The listing builds one solid part. Answer for the finished solid, in the listing's coordinates (mm). A direction names the side the tool comes from. Give positions to 0.01 mm unless a question says otherwise; leave off trailing zeros. Write each loop counter-clockwise with the first axis right and the second up, starting at its lowest first coordinate (ties: lowest second). Pieces come first, ordered by that corner, then holes. Notation, with made-up numbers: (-24.75, 46.5) - (9.25, 46.5) arc R17 cw to (9.25, 64.5) - close; hole circle Ø10 at (-4, 25.25). An arc over 180 degrees is marked (long way). Answer as CSV lines item,"result". Start each with the question number.
(1) For a pull along X with two mould halves and no side action, classify faces 5 (the face through (2, 3, 0)), 6 (the face through (20, 2, 0)), 7 (the face through (10, 0, 0)) as pulls with the +X half, pulls with the -X half, needs draft (parallel to the pull), parting line crosses it, or undercut.
(2) Straight lines are drawn through the part: probe 1 along X at (y, z) = (2.5, 0.8); probe 2 along Y at (x, z) = (2.75, 0.45); probe 3 along Z at (x, y) = (1.5, 5.2). For each, find the intervals that lie inside material, in ascending order.
(3) Find section C-C (x = 7.5). Write down the section's boundary in (y, z).
(4) Find section D-D (y = 2.7). Write down the section's boundary in (x, z).
(5) Each of these flat-tipped pins is pushed along its axis until it touches: pin 1 Ø1 at (y, z) = (4, 0.5) entering from -X; pin 2 Ø0.8 at (x, z) = (19.5, -1.5) entering from +Y; pin 3 Ø0.8 at (x, y) = (1, 4.5) entering from +Z; pin 4 Ø1.2 at (x, y) = (19, 5) entering from -Z. Where does it stop, or does it pass through?
(6) Find section B-B (z = 0.15). Write down the section's boundary in (x, y).
(7) For faces 1 (the face through (1, 4, 1.5)), 2 (the face through (18, 3, 0)), 3 (the face through (1, 5, -1)), 4 (the face through (10, 1, 2)), determine the directions among +Z, -Z, +X, -X, +Y, -Y from which every point of the face is accessible in a straight line to the end or side of a thin tool.
(8) Find section A-A (y = 5.1). Write down the section's boundary in (x, z), then the cut area to 3 significant figures.
from build123d import *

# Parameters (mm, degrees)
BOSS_EXTRUDE1_DEPTH      = 2
BOSS_EXTRUDE1_DEPTH_BACK = 2
SKETCH2_W                = 1
SKETCH2_H                = 1.5
CUT_EXTRUDE1_DEPTH       = 21.838665984


with BuildPart() as part:
    # Sketch1 → Boss-Extrude1 (new, two sides: drawn at the far end of the back side and taken through both)
    with BuildSketch(Plane.XY.offset(-BOSS_EXTRUDE1_DEPTH_BACK)):
        Polygon((2, 2), (18, 2), (18, 5.5), (20, 5.5), (20, 0), (0, 0), (0, 5.5), (2, 5.5), align=None)
    extrude(amount=BOSS_EXTRUDE1_DEPTH + BOSS_EXTRUDE1_DEPTH_BACK)

    # Sketch2 → Cut-Extrude1 (cut, symmetric)
    with BuildSketch(Plane.ZY):
        with Locations((-1.5, 4.75)):
            Rectangle(SKETCH2_W, SKETCH2_H)
    cut_extrude1 = extrude(amount=CUT_EXTRUDE1_DEPTH, both=True, mode=Mode.SUBTRACT)

    # Mirror1: Cut-Extrude1 across plane
    add(cut_extrude1.mirror(Plane.XY), mode=Mode.SUBTRACT)


solid = part.part
Result set:
1,face 5,"undercut"
1,face 6,"pulls with the +X half"
1,face 7,"needs draft"
2,probe 1,"0 to 2, 18 to 20"
2,probe 2,"0 to 2"
2,probe 3,"-1 to 1"
3,outline,"(0, -2) - (2, -2) - (2, 2) - (0, 2) - close"
4,outline,"(0, -2) - (2, -2) - (2, 2) - (0, 2) - close; (18, -2) - (20, -2) - (20, 2) - (18, 2) - close"
5,pin 1,"x = 0"
5,pin 2,"y = 4"
5,pin 3,"z = 1"
5,pin 4,"z = -1"
6,outline,"(0, 0) - (20, 0) - (20, 5.5) - (18, 5.5) - (18, 2) - (2, 2) - (2, 5.5) - (0, 5.5) - close"
7,face 1,"+Z, +X, -X, +Y"
7,face 2,"+Z, -Z, +Y"
7,face 3,"-Z, +X, -X, +Y"
7,face 4,"+Z, +X, -X, +Y, -Y"
8,outline,"(0, -1) - (2, -1) - (2, 1) - (0, 1) - close; (18, -1) - (20, -1) - (20, 1) - (18, 1) - close"
8,area,"8.00 mm^2"
